Input: part model. Units: mm. Frame: model coordinates. Coordinates: 2 decimals unless noted, no trailing zeros. Write each loop counter-clockwise with the first axis right and the second up, starting at its lowest first coordinate (ties: lowest second). Pieces come first, ordered by that corner, then holes. Notation, with made-up numbers: M 28,82.5 L 56,82.5 A24 ccw 56,120.5 Z; hole C 69.25,-30.75 d6. An arc over 180 degrees is marked long. Answer as a JSON object with one key per item and string values. Group by question number.
Autodesk Inventor part; units mm, degrees
ref_plane "YZ Plane" through (0, 0, 0) normal (1, 0, 0) x (0, 1, 0)
ref_plane "XZ Plane" through (0, 0, 0) normal (0, 1, 0) x (-1, 0, 0)
ref_plane "XY Plane" through (0, 0, 0) normal (0, 0, 1) x (1, 0, 0)
sketch "Sketch1" plane through (0, 0, 0) normal (0, 1, 0) x (-1, 0, 0)
  line L0 (0, 0) -> (0, -71.8312)
  line L1 (0, 0) -> (159.893, -71.189)
  line L2 (159.893, -71.189) -> (159.893, -143.0202)
  line L3 (159.893, -143.0202) -> (0, -71.8312)
  circle A0 centre (96.393, -74.364) radius 14.2875
  line L4 (0, -71.8312) -> (27.94, -99.7712)
  line L5 (27.94, -99.7712) -> (159.893, -143.0202)
  point P0 (38.467, -74.3966)
  dimension "d0" = 71.8312
  dimension "d1" = 66
  dimension "d2" = 159.893
  dimension "d4" = 71.8312
  dimension "d5" = 3.175
  dimension "d6" = 63.5
  dimension "d7" = 28.575
  dimension "d10" = 38.467
  dimension "d11" = 74.3966
  dimension "d12" = 27.94
  dimension "d14" = 21
extrude "Extrusion1" add sketch "Sketch1" along normal blind 3.175 contours L1 L2 L3 L0
extrude "Extrusion3" add sketch "Sketch1" along normal blind 3.175 contours L3 L5 L4
hole "Hole2" at (-96.393, 0, -74.364) at (-38.467, 0, -74.3966) direction (0, 1, 0) diameter 28.575 end through all
properties part number "StorageGusset.ver1-1111-2020"
Q1. Section C-C, the plane y = 0.8. Return the cut outline in (x, z) (1 decimal).
Q2. Section D-D, the plane x = -32.5. Return the cut outline in (y, z) (3 decimals).
Q3. Section A-A, the plane z = -84. Return the cut outline in (x, y) (3 decimals).
Q4. Pin query (flat end, axial travel): pin 1 Ø1 at (x, y) = (-72, 0.5) entering from -Z; pin 2 Ø1.5 at (x, y) = (-47.5, 3) entering from -Z. Return the tip coordinate at first contact, or that it passes through.
Q5. Line query: line 1 (X direction, y = 1.1, z = -77.5); line 2 (X direction, y = 1.2, z = -82); line 3 (Z direction, x = -25.5, y = 0.3). Output: solid intervals per line, ascending. Write a range as from..to.
Q6. Draft query along Z for faces 1 (the flat face through (-13.774, 1.565, -85.606)), 2 (the flat face through (-78.827, 1.565, -35.096)), 3 (the cylindrical face through (-32.995, 1.61, -87.595)). Return one class per face: released by +Z, released by -Z, zero draft, split by the parting line, or undercut.
Q7. Section B-B, the plane x = -99.5. Return the cut outline in (y, z) (3 decimals), and give its area (3 significant figures).
Filled in:
{
 "1": {"outline": "M -159.9,-143 L -27.9,-99.8 L 0,-71.8 L 0,0 L -159.9,-71.2 Z; hole C -96.4,-74.4 d28.6; hole C -38.5,-74.4 d28.6"},
 "2": {"outline": "M 0,-101.266 L 3.175,-101.266 L 3.175,-87.378 L 0,-87.378 Z; M 0,-61.415 L 3.175,-61.415 L 3.175,-14.47 L 0,-14.47 Z"},
 "3": {"outline": "M -159.893,0 L -106.942,0 L -106.942,3.175 L -159.893,3.175 Z; M -85.844,0 L -49.046,0 L -49.046,3.175 L -85.844,3.175 Z; M -27.888,0 L -12.169,0 L -12.169,3.175 L -27.888,3.175 Z"},
 "4": {"pin 1": "z = -114.38", "pin 2": "z = -106.43"},
 "5": {"line 1": "-159.89..-110.33, -82.45..-52.41, -24.52..-5.67", "line 2": "-159.89..-108.47, -84.32..-50.56, -26.37..-10.17", "line 3": "-97.33..-80.4, -68.4..-11.35"},
 "6": {"face 1": "released by -Z", "face 2": "released by +Z", "face 3": "undercut"},
 "7": {"outline": "M 0,-123.226 L 3.175,-123.226 L 3.175,-88.31 L 0,-88.31 Z; M 0,-60.418 L 3.175,-60.418 L 3.175,-44.3 L 0,-44.3 Z", "area": "162 mm^2"}
}
